Input: part model. Units: mm. Frame: model coordinates. Face numbers are marked on the shaded views. A direction names the side the tool comes from. Give positions to 0.01 mm unless a question says otherwise; leave off trailing zeros. Loops run counter-clockwise (first coordinate to the right, second up) from the corner with the lowest first, then second, coordinate; pieces in that order, holes last. Notation, with made-up numbers: (17.25, 51) - (55.25, 51) arc R18 ccw to (55.25, 73) - close; hole circle Ø8 at (40.25, -24). An arc over 180 degrees is marked (long way). One line per question, with ' | ' between items. Start each with the question number.
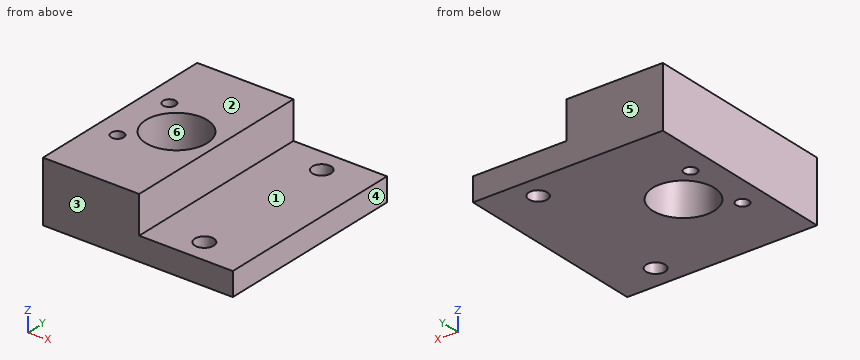
from build123d import *

# Parameters (mm, degrees)
F0_W     = 20
F0_H     = 42
F0_R     = 2.0193883272
F0_R_2   = 2
F1_DEPTH = 5
F0_W_2   = 20.55
F0_R_3   = 1.35
F0_R_4   = 6.55
F2_DEPTH = 13


# Not quite as in the source:
# - a feature of the source that left no trace in its solid (it failed there, or was rolled back) is left out


with BuildPart() as f1:
    # F0 (on Top) → F1 (new body)
    with BuildSketch(Plane.XY):
        with Locations((13.4585087977, 14.1658929903)):
            Rectangle(F0_W, F0_H)
        with Locations((13.4585087977, -1.8341070097)):
            Circle(F0_R, mode=Mode.SUBTRACT)
        with Locations((13.4585087977, 30.1658929903)):
            Circle(F0_R_2, mode=Mode.SUBTRACT)
    extrude(amount=F1_DEPTH)

    # F0 (on Top) → F2 (join)
    with BuildSketch(Plane.XY):
        with Locations((-6.8164912023, 14.1658929903)):
            Rectangle(F0_W_2, F0_H)
        with Locations((-12.1125590142, 7.0948251784)):
            Circle(F0_R_3, mode=Mode.SUBTRACT)
        with Locations((-5.0414912023, 14.1658929903)):
            Circle(F0_R_4, mode=Mode.SUBTRACT)
        with Locations((-12.1125590142, 21.2369608022)):
            Circle(F0_R_3, mode=Mode.SUBTRACT)
    extrude(amount=F2_DEPTH)


solid = f1.part
Q1. Section B-B, the plane z = 3.75. Output: boundary loops of the cut face in (x, y).
Q2. Section A-A, the plane y = 11.5. Output: boundary loops of the cut face in (x, z).
Q3. Draft query along Y for the marked faces 3, 4, 5 and 6. Return one class per face: +Y half, -Y half, draft (parallel to the pull), parting line (faces both ways), or undercut.
Q4. Section D-D, the plane z = 9.25. Output: boundary loops of the cut face in (x, y), plus the area to 3 significant figures.
Q5. Access query for the marked faces 1 and 2. Directions: +Z, -Z, +X, -X, +Y, -Y. A direction counts if a zero-diameter tool reaches every point of the face in a straight line with its end or side. Return the directions, or none.
Q6. Section C-C, the plane x = -3. Output: boundary loops of the cut face in (y, z).
Q7. Line query: L1, parallel to X at y = 20, z = 7.75; L2, parallel to Y at x = -5, z = 0.5; L3, parallel to Z at x = 5.5, y = -5. Output: solid intervals per line, ascending. Write a range as from..to.
Q8. First-contact query: pin 1 (1.5 mm diameter, centred on x = -11, y = 21.5, fed in from +Z); pin 2 (3.5 mm diameter, centred on x = 13.46, y = 30.17, fed in from -Z); pin 3 (1.5 mm diameter, centred on y = 9, z = 8.5, fed in from +X); pin 4 (16 mm diameter, centred on x = 14.5, y = 20.5, fed in from +Z). Flat tips, straight axial feed; report the tip coordinate or a pass-through.
Solved:
1) outline: (-17.09, -6.83) - (23.46, -6.83) - (23.46, 35.17) - (-17.09, 35.17) - close; hole circle Ø2.7 at (-12.11, 7.09); hole circle Ø2.7 at (-12.11, 21.24); hole circle Ø13.1 at (-5.04, 14.17); hole circle Ø4.04 at (13.46, -1.83); hole circle Ø4 at (13.46, 30.17)
2) outline: (-17.09, 0) - (-11.02, 0) - (-11.02, 13) - (-17.09, 13) - close; (0.94, 0) - (23.46, 0) - (23.46, 5) - (3.46, 5) - (3.46, 13) - (0.94, 13) - close
3) face 3: -Y half | face 4: draft | face 5: +Y half | face 6: undercut
4) outline: (-17.09, -6.83) - (3.46, -6.83) - (3.46, 35.17) - (-17.09, 35.17) - close; hole circle Ø2.7 at (-12.11, 7.09); hole circle Ø2.7 at (-12.11, 21.24); hole circle Ø13.1 at (-5.04, 14.17) | area: 717 mm²
5) face 1: +Z, +X, +Y, -Y | face 2: +Z, +X, -X, +Y, -Y
6) outline: (-6.83, 0) - (7.94, 0) - (7.94, 13) - (-6.83, 13) - close; (20.39, 0) - (35.17, 0) - (35.17, 13) - (20.39, 13) - close
7) L1: x = -17.09..-12.65, -11.57..-8.02, -2.06..3.46 | L2: y = -6.83..7.62, 20.72..35.17 | L3: z = 0..5
8) pin 1: stops at z = 13 | pin 2: passes through | pin 3: stops at x = 3.46 | pin 4: stops at z = 5
